CAD build for the part. Positions are in the model's coordinates, mm. Give positions to 0.01 mm unless a question says otherwise; leave off trailing zeros. Use one line per item in the form item = value.
```python
from build123d import *

# Parameters (mm, degrees)
SKETCH2_W               = 63.5
SKETCH2_H               = 36.83
BOSS_EXTRUDE1_DEPTH     = 17.78
SKETCH3_R               = 1.25
CUT_EXTRUDE1_DEPTH      = 1
CUT_EXTRUDE1_DEPTH_BACK = 36.56


with BuildPart() as part:
    # Sketch2 → Boss-Extrude1 (new body, symmetric)
    with BuildSketch(Plane(origin=(0, 0, 0), x_dir=(1, 0, 0), z_dir=(0, 1, 0))):
        Rectangle(SKETCH2_W, SKETCH2_H)
    extrude(amount=BOSS_EXTRUDE1_DEPTH, both=True)

    # Sketch3 → Cut-Extrude1 (cut, two sides)
    with BuildSketch(Plane(origin=(0, 17.78, 0), x_dir=(1, 0, 0), z_dir=(0, 1, 0))) as cut_extrude1_sk:
        with Locations((-28.88075, 15.64005)):
            Circle(SKETCH3_R)
        with Locations((28.88075, 15.64005)):
            Circle(SKETCH3_R)
        with Locations((28.88075, -15.64005)):
            Circle(SKETCH3_R)
        with Locations((-28.88075, -15.64005)):
            Circle(SKETCH3_R)
    extrude(amount=CUT_EXTRUDE1_DEPTH, mode=Mode.SUBTRACT)
    extrude(cut_extrude1_sk.sketch, amount=-CUT_EXTRUDE1_DEPTH_BACK, mode=Mode.SUBTRACT)


solid = part.part
```
1. Mould opens along Z. For faces 1 (the flat face through (0, 0, 18.415)), 2 (the flat face through (0, -17.78, 0)), 3 (the cylindrical face through (28.72, 0.25, 14.4)), 4 (the cylindrical face through (-27.726, 0.249, -15.161)) say: pulls with the +Z half, pulls with the -Z half, needs draft (parallel to the pull), parting line crosses it, or undercut.
Result sheet:
face_1 = pulls with the +Z half
face_2 = needs draft
face_3 = undercut
face_4 = undercut
2. Drill centre lines: line 1 (Z direction, x = -29, y = 8.5) (3 decimals); line 2 (X direction, y = 3, z = 15.5); line 3 (Z direction, x = 28, y = 6.5) (3 decimals). Where is each one in solid material? Low to high.
Result sheet:
line_1 = -18.415 to -16.884, -14.396 to 14.396, 16.884 to 18.415
line_2 = -31.75 to -30.12, -27.64 to 27.64, 30.12 to 31.75
line_3 = -18.415 to -16.527, -14.753 to 14.753, 16.527 to 18.415
3. Drop a flat-ended pin along its axis: P1, Ø3, axis at x = 28.88, z = -15.64, coming from the -Y side. Give the stop position or say it passes through.
Result sheet:
P1 = -17.78
